Read the model definition and answer for the solid it produces. Units are mm, in the model's axes. Face numbers are marked on the shaded views. A direction names the side the tool comes from. Coordinates: 2 decimals unless noted, no trailing zeros. Loops run counter-clockwise (first coordinate to the right, second up) from the corner with the lowest first, then second, coordinate; pieces in that order, holes last. Notation, with made-up numbers: M -2.5,-38.5 L 44.5,-38.5 A18 ccw 44.5,-13.5 Z; hole C 62.25,-17 d3. An arc over 180 degrees is marked long. Use one line per item in the form item = value. Start each with the question number.
1. For a pull along X with two mould halves and no side action, classify the marked faces 4, 5 and 6 as released by +X, released by -X, zero draft, split by the parting line, or undercut.
2. Find the intervals of material crossed by probe 1 along X at (y, z) = (6.8, -65); probe 2 along Z at (x, y) = (-13, 1.75); probe 3 along X at (y, z) = (9.4, -65), in increasing order. Write a range as [from, to].
3. The part is cut by section A-A (z = 15). Give the vertices of the cut face in (x, y), plus the area to 3 significant figures.
4. The part is cut by section C-C (x = 9). Give the number of separate pieces and of enclosed holes in the cut face, plus the area to 3 significant figures.
5. A tool of negligible diameter and unlimited length cuts with its end or side. For the marked faces 1, 2 and 3, from which of +Z, -Z, +X, -X, +Y, -Y can it reach the whole face along a straight path? Write none if from no direction.
6. The part is cut by section D-D (y = 0). Give the vertices of the cut face in (x, z).
7. Flat-ended cylindrical pins translate along their axes: pin 1 (5.5 mm diameter, centred on x = -16, z = 15, fed in from -Y); pin 2 (5 mm diameter, centred on y = 13.5, z = -38.5, fed in from +X); pin 3 (1 mm diameter, centred on x = 13, z = -41.5, fed in from -Y); pin 4 (4.5 mm diameter, centred on y = 11, z = -31, fed in from -X). Find the tip coordinate at first contact, or state that the pin passes through.
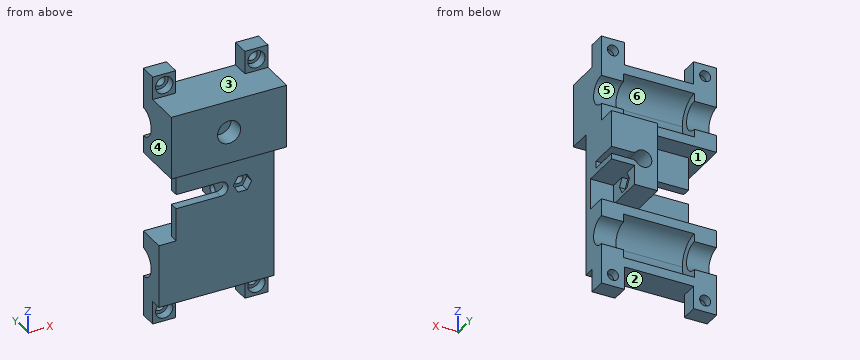
from build123d import *

# Parameters (mm, degrees)
SKETCH1_W                  = 40
SKETCH1_H                  = 22
BOSS_EXTRUDE1_DEPTH        = 11
SKETCH2_W                  = 40
SKETCH2_H                  = 22
SKETCH2_R                  = 4
BOSS_EXTRUDE2_DEPTH        = 7
SKETCH3_W                  = 24.5
SKETCH3_H                  = 15.5
CUT_EXTRUDE1_DEPTH         = 7.75
FILLET1_R                  = 7.75
SKETCH4_R                  = 5
CUT_EXTRUDE2_DEPTH         = 36.805900352
SKETCH5_W                  = 8
SKETCH5_H                  = 8
SKETCH5_R                  = 1.905800151
BOSS_EXTRUDE3_DEPTH        = 6
CUT_EXTRUDE3_START         = -3
SKETCH6_R                  = 3
SKETCH6_R_2                = 1.905800151
CUT_EXTRUDE3_DEPTH         = 3
SKETCH7_W                  = 16
SKETCH7_H                  = 16.5
BOSS_EXTRUDE5_DEPTH        = 28
MIRROR14_COPY_1_SKETCH_W   = 8
MIRROR14_COPY_1_SKETCH_H   = 8
MIRROR14_COPY_1_SKETCH_R   = 1.905800151
MIRROR14_COPY_1_DEPTH      = 6
MIRROR14_START             = -3
MIRROR14_COPY_2_SKETCH_R   = 3
MIRROR14_COPY_2_SKETCH_R_2 = 1.905800151
MIRROR14_COPY_2_DEPTH      = 3
FILLET1_OF_MIRROR14_R      = 7.75
SKETCH9_W                  = 28
SKETCH9_H                  = 3
BOSS_EXTRUDE6_DEPTH        = 18
CUT_EXTRUDE4_DEPTH         = 10
CUT_EXTRUDE5_DEPTH         = 74.288812243
CUT_EXTRUDE5_DEPTH_BACK    = 74.288812243
SKETCH11_R                 = 1.75
CUT_EXTRUDE6_DEPTH         = 76.121568141
CUT_EXTRUDE6_DEPTH_BACK    = 76.121568141
SKETCH12_R                 = 1.75
FILLET2_R                  = 2
CUT_EXTRUDE12_START        = -3
SKETCH17_R                 = 1.75
CUT_EXTRUDE12_DEPTH        = 3
CUT_EXTRUDE13_DEPTH        = 74.097537578
CUT_EXTRUDE13_DEPTH_BACK   = 74.097537578
SKETCH18_W                 = 18
SKETCH18_H                 = 5
FILLET3_R                  = 2.5
CUT_EXTRUDE14_DEPTH        = 74.710582687
CUT_EXTRUDE15_START        = -10
SKETCH21_R                 = 1.75
CUT_EXTRUDE15_DEPTH        = 10
SKETCH20_W                 = 36.163748027
SKETCH20_H                 = 4
CUT_EXTRUDE16_DEPTH        = 13.5
SKETCH22_W                 = 6.75
SKETCH22_H                 = 13.5
CUT_EXTRUDE18_DEPTH        = 8
SKETCH23_R                 = 4
BOSS_EXTRUDE8_DEPTH        = 1


with BuildPart() as part:
    # Sketch1 → Boss-Extrude1 (new body)
    with BuildSketch(Plane(origin=(0, 0, 0), x_dir=(1, 0, 0), z_dir=(0, 1, 0))):
        Rectangle(SKETCH1_W, SKETCH1_H)
    boss_extrude1 = extrude(amount=BOSS_EXTRUDE1_DEPTH)

    # Sketch2 → Boss-Extrude2 (add)
    with BuildSketch(Plane(origin=(0, 0, 0), x_dir=(1, 0, 0), z_dir=(0, 1, 0))):
        Rectangle(SKETCH2_W, SKETCH2_H)
        with Locations(Location((0, 0, 0), (0, 0, 270))):
            Circle(SKETCH2_R, mode=Mode.SUBTRACT)
    boss_extrude2 = extrude(amount=-BOSS_EXTRUDE2_DEPTH)

    # Sketch3 → Cut-Extrude1 (cut)
    with BuildSketch(Plane(origin=(0, 11, 0), x_dir=(1, 0, 0), z_dir=(0, 1, 0))):
        Rectangle(SKETCH3_W, SKETCH3_H)
    cut_extrude1 = extrude(amount=-CUT_EXTRUDE1_DEPTH, mode=Mode.SUBTRACT)

    # Fillet1
    fillet1_edges = [part.edges().sort_by_distance(p)[0] for p in [
        (0, 3.25, 7.75),
        (0, 3.25, -7.75),
    ]]
    fillet(fillet1_edges, radius=FILLET1_R - 0.0001)  # a hair under: the kernel refuses the full size

    # Sketch4 → Cut-Extrude2 (cut, symmetric)
    with BuildSketch(Plane(origin=(-12.25, 0, 0), x_dir=(0, 0, -1), z_dir=(1, 0, 0))):
        with Locations((0, 11)):
            Circle(SKETCH4_R)
    cut_extrude2 = extrude(amount=CUT_EXTRUDE2_DEPTH, both=True, mode=Mode.SUBTRACT)

    # Sketch5 → Boss-Extrude3 (add)
    with BuildSketch(Plane(origin=(0, 11, 0), x_dir=(1, 0, 0), z_dir=(0, 1, 0))):
        with Locations((16, -15)):
            Rectangle(SKETCH5_W, SKETCH5_H)
        with Locations(Location((16, -15, 0), (0, 0, 270))):
            Circle(SKETCH5_R, mode=Mode.SUBTRACT)
    boss_extrude3 = extrude(amount=-BOSS_EXTRUDE3_DEPTH)

    # Sketch6 → Cut-Extrude3 (cut)
    with BuildSketch(Plane.XZ.offset(-5).offset(CUT_EXTRUDE3_START)):
        with Locations(Location((16, 15, 0), (0, 0, 270))):
            Circle(SKETCH6_R)
        with Locations(Location((16, 15, 0), (0, 0, 90))):
            Circle(SKETCH6_R_2, mode=Mode.SUBTRACT)
    cut_extrude3 = extrude(amount=CUT_EXTRUDE3_DEPTH, mode=Mode.SUBTRACT)

    # Mirror8: Boss-Extrude3, Cut-Extrude3 across plane
    add(boss_extrude3.mirror(Plane(origin=(0, 0, 0), x_dir=(0, 0, 1), z_dir=(1, 0, 0))))
    add(cut_extrude3.mirror(Plane(origin=(0, 0, 0), x_dir=(0, 0, 1), z_dir=(1, 0, 0))), mode=Mode.SUBTRACT)

    # Sketch7 → Boss-Extrude5 (add)
    with BuildSketch(Plane(origin=(0, 0, -11), x_dir=(-1, 0, 0), z_dir=(0, 0, -1))):
        with Locations((-12, 9.25)):
            Rectangle(SKETCH7_W, SKETCH7_H)
    extrude(amount=BOSS_EXTRUDE5_DEPTH)

    # Mirror14: Boss-Extrude1, Boss-Extrude2, Cut-Extrude1, Cut-Extrude2, Boss-Extrude3, Cut-Extrude3 across plane
    add(boss_extrude1.mirror(Plane.XY.offset(-25)))
    add(boss_extrude2.mirror(Plane.XY.offset(-25)))
    add(cut_extrude1.mirror(Plane.XY.offset(-25)), mode=Mode.SUBTRACT)
    add(cut_extrude2.mirror(Plane.XY.offset(-25)), mode=Mode.SUBTRACT)
    add(boss_extrude3.mirror(Plane.XY.offset(-25)))
    add(cut_extrude3.mirror(Plane.XY.offset(-25)), mode=Mode.SUBTRACT)

    # Mirror14 copy 1 sketch → Mirror14 copy 1 (add)
    with BuildSketch(Plane(origin=(0, 11, -50), x_dir=(-1, 0, 0), z_dir=(0, 1, 0))):
        with Locations((16, -15)):
            Rectangle(MIRROR14_COPY_1_SKETCH_W, MIRROR14_COPY_1_SKETCH_H)
        with Locations(Location((16, -15, 0), (0, 0, 270))):
            Circle(MIRROR14_COPY_1_SKETCH_R, mode=Mode.SUBTRACT)
    extrude(amount=-MIRROR14_COPY_1_DEPTH)

    # Mirror14 copy 2 sketch → Mirror14 copy 2 (cut)
    with BuildSketch(Plane(origin=(0, 5, -50), x_dir=(-1, 0, 0), z_dir=(0, -1, 0)).offset(MIRROR14_START)):
        with Locations(Location((16, 15, 0), (0, 0, 270))):
            Circle(MIRROR14_COPY_2_SKETCH_R)
        with Locations(Location((16, 15, 0), (0, 0, 90))):
            Circle(MIRROR14_COPY_2_SKETCH_R_2, mode=Mode.SUBTRACT)
    extrude(amount=MIRROR14_COPY_2_DEPTH, mode=Mode.SUBTRACT)

    # Fillet1 of Mirror14
    fillet1_of_mirror14_edges = [part.edges().sort_by_distance(p)[0] for p in [
        (0, 3.25, -57.75),
        (0, 3.25, -42.25),
    ]]
    fillet(fillet1_of_mirror14_edges, radius=FILLET1_OF_MIRROR14_R - 0.0001)  # a hair under: the kernel refuses the full size

    # Sketch9 → Boss-Extrude6 (add)
    with BuildSketch(Plane.ZY.offset(-4)):
        with Locations((-25, 2.5)):
            Rectangle(SKETCH9_W, SKETCH9_H)
    extrude(amount=BOSS_EXTRUDE6_DEPTH)

    # Sketch10 → Cut-Extrude4 (cut)
    with BuildSketch(Plane(origin=(0, 17.5, 0), x_dir=(1, 0, 0), z_dir=(0, 1, 0))):
        with BuildLine():
            Line((9, 26.25), (9, 23.75))
            Line((9, 23.75), (11.727178029, 23.75))
            ThreePointArc((11.727178029, 23.75), (11.931001031, 24.360286817), (12, 25))
            ThreePointArc((12, 25), (11.931001031, 25.639713183), (11.727178029, 26.25))
            Line((11.727178029, 26.25), (9, 26.25))
        make_face()
        with BuildLine():
            Line((11.727178029, 23.75), (9, 23.75))
            Line((9, 23.75), (9, 26.25))
            Line((9, 26.25), (11.727178029, 26.25))
            ThreePointArc((11.727178029, 26.25), (6, 25), (11.727178029, 23.75))
        make_face()
        with BuildLine():
            ThreePointArc((12, 25), (11.931001031, 24.360286817), (11.727178029, 23.75))
            Line((11.727178029, 23.75), (20, 23.75))
            Line((20, 23.75), (20, 26.25))
            Line((20, 26.25), (11.727178029, 26.25))
            ThreePointArc((11.727178029, 26.25), (11.931001031, 25.639713183), (12, 25))
        make_face()
    extrude(amount=-CUT_EXTRUDE4_DEPTH, mode=Mode.SUBTRACT)

    # Sketch11 → Cut-Extrude5 (cut, two sides: drawn at the far end of the back side and taken through both)
    with BuildSketch(Plane(origin=(0, 7.5, 0), x_dir=(1, 0, 0), z_dir=(0, 1, 0)).offset(-CUT_EXTRUDE5_DEPTH_BACK)):
        with Locations(Location((9, 25, 0), (0, 0, 270))):
            Circle(SKETCH11_R)
    extrude(amount=CUT_EXTRUDE5_DEPTH + CUT_EXTRUDE5_DEPTH_BACK, mode=Mode.SUBTRACT)

    # Sketch12 → Cut-Extrude6 (cut, two sides: drawn at the far end of the back side and taken through both)
    with BuildSketch(Plane.ZY.offset(-4).offset(-CUT_EXTRUDE6_DEPTH_BACK)):
        with Locations((-31, 11)):
            Circle(SKETCH12_R)
    extrude(amount=CUT_EXTRUDE6_DEPTH + CUT_EXTRUDE6_DEPTH_BACK, mode=Mode.SUBTRACT)

    # Fillet2
    fillet2_edges = [part.edges().sort_by_distance(p)[0] for p in [
        (11.727178029, 12.5, -23.75),
        (11.727178029, 12.5, -26.25),
    ]]
    fillet(fillet2_edges, radius=FILLET2_R)

    # Sketch17 → Cut-Extrude12 (cut)
    with BuildSketch(Plane.XZ.offset(-1).offset(CUT_EXTRUDE12_START)):
        Polygon((12.175426481, -25), (10.58771324, -22.25), (7.41228676, -22.25), (5.824573519, -25), (7.41228676, -27.75), (10.58771324, -27.75), align=None)
        with Locations(Location((9, -25, 0), (0, 0, 90))):
            Circle(SKETCH17_R, mode=Mode.SUBTRACT)
    extrude(amount=CUT_EXTRUDE12_DEPTH, mode=Mode.SUBTRACT)

    # Sketch18 → Cut-Extrude13 (cut, two sides: drawn at the far end of the back side and taken through both)
    with BuildSketch(Plane(origin=(0, 4, 0), x_dir=(1, 0, 0), z_dir=(0, 1, 0)).offset(-CUT_EXTRUDE13_DEPTH_BACK)):
        with Locations((-5, 25)):
            Rectangle(SKETCH18_W, SKETCH18_H)
    extrude(amount=CUT_EXTRUDE13_DEPTH + CUT_EXTRUDE13_DEPTH_BACK, mode=Mode.SUBTRACT)

    # Fillet3
    fillet3_edges = [part.edges().sort_by_distance(p)[0] for p in [
        (4, 2.5, -27.5),
        (4, 2.5, -22.5),
    ]]
    fillet(fillet3_edges, radius=FILLET3_R - 0.0001)  # a hair under: the kernel refuses the full size

    # Sketch19 → Cut-Extrude14 (cut, through all)
    with BuildSketch(Plane.XZ.offset(-1)):
        Polygon((20, -61), (20, -39), (-14, -39), (-20, -39), (-20, -61), align=None)
    extrude(amount=CUT_EXTRUDE14_DEPTH, mode=Mode.SUBTRACT)

    # Sketch21 → Cut-Extrude15 (cut)
    with BuildSketch(Plane(origin=(20, 0, 0), x_dir=(0, 0, -1), z_dir=(1, 0, 0)).offset(CUT_EXTRUDE15_START)):
        Polygon((31, 14.175426481), (28.25, 12.58771324), (28.25, 9.41228676), (31, 7.824573519), (33.75, 9.41228676), (33.75, 12.58771324), align=None)
        with Locations((31, 11)):
            Circle(SKETCH21_R, mode=Mode.SUBTRACT)
    extrude(amount=CUT_EXTRUDE15_DEPTH, mode=Mode.SUBTRACT)

    # Sketch20 → Cut-Extrude16 (cut)
    with BuildSketch(Plane(origin=(0, 17.5, 0), x_dir=(1, 0, 0), z_dir=(0, 1, 0))):
        with Locations((22.081874014, 37)):
            Rectangle(SKETCH20_W, SKETCH20_H)
    extrude(amount=-CUT_EXTRUDE16_DEPTH, mode=Mode.SUBTRACT)

    # Sketch22 → Cut-Extrude18 (cut)
    with BuildSketch(Plane(origin=(20, 0, 0), x_dir=(0, 0, -1), z_dir=(1, 0, 0))):
        with Locations((31.625, 10.75)):
            Rectangle(SKETCH22_W, SKETCH22_H)
    extrude(amount=-CUT_EXTRUDE18_DEPTH, mode=Mode.SUBTRACT)

    # Sketch23 → Boss-Extrude8 (add)
    with BuildSketch(Plane.XZ):
        with Locations(Location((0, 0, 0), (0, 0, 90))):
            Circle(SKETCH23_R)
    extrude(amount=BOSS_EXTRUDE8_DEPTH)


solid = part.part
Computed values:
q1.face_4 = released by -X
q1.face_5 = zero draft
q1.face_6 = undercut
q2.probe_1 = [-20, -19], [-13, -12], [12, 13], [19, 20]
q2.probe_2 = [-61, -27.5], [-22.5, 11]
q2.probe_3 = [-20, -17.91], [-14.09, -12], [12, 14.09], [17.91, 20]
q3.outline = M -20,5 L -19,5 L -19,8 L -17.91,8 L -17.91,11 L -20,11 Z; M -14.09,8 L -13,8 L -13,5 L -12,5 L -12,11 L -14.09,11 Z; M 12,5 L 13,5 L 13,8 L 14.09,8 L 14.09,11 L 12,11 Z; M 17.91,8 L 19,8 L 19,5 L 20,5 L 20,11 L 17.91,11 Z
q3.area = 37.1 mm²
q4.separate_pieces = 2
q4.enclosed_holes = 1
q4.area = 737 mm²
q5.face_1 = -X
q5.face_2 = -Z, -Y
q5.face_3 = +Z, -Y
q6.outline = M -20,-11 L 20,-11 L 20,11 L -20,11 Z
q7.pin_1 = 8
q7.pin_2 = through
q7.pin_3 = 1
q7.pin_4 = 4
